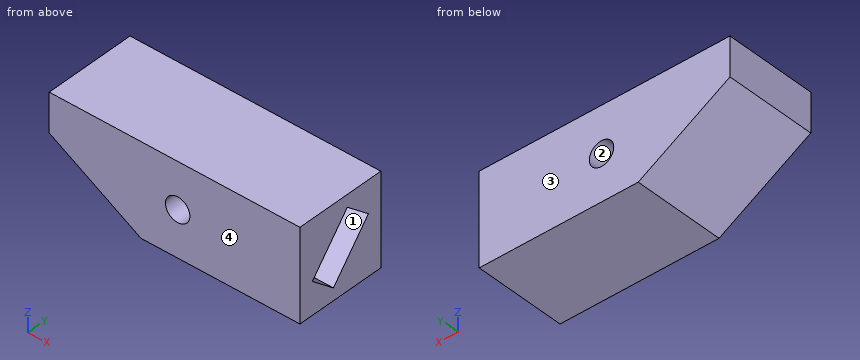
```python
from build123d import *

# Parameters (mm, degrees)
EXTRUDE_1_DEPTH     = 30
SKETCH_2_R          = 4
CUT_EXTRUDE_1_DEPTH = 49.476798574
CUT_EXTRUDE_4_DEPTH = 25
SKETCH1_W           = 30
SKETCH1_H           = 30
BOSS_EXTRUDE1_DEPTH = 27
CHAMFER1_SIZE       = 30
CHAMFER1_SIZE2      = 17.320508076


with BuildPart() as part:
    # Эскиз1 → Бобышка-Вытянуть1 (new body)
    with BuildSketch(Plane(origin=(0, 0, 0), x_dir=(1, 0, 0), z_dir=(0, 1, 0))):
        Polygon((-20, -15), (-35, -15), (-35, 15), (-20, 15), (20, 15), (20, -15), align=None)
    extrude(amount=EXTRUDE_1_DEPTH)

    # Эскиз2 → Вырез-Вытянуть1 (cut, through all)
    with BuildSketch(Plane(origin=(0, 30, 0), x_dir=(1, 0, 0), z_dir=(0, 1, 0))):
        with Locations(Location((-20, 0, 0), (0, 0, 270))):
            Circle(SKETCH_2_R)
    extrude(amount=-CUT_EXTRUDE_1_DEPTH, mode=Mode.SUBTRACT)

    # Эскиз5 → Вырез-Вытянуть4 (cut)
    with BuildSketch(Plane(origin=(20, 0, 0), x_dir=(0, 0, -1), z_dir=(1, 0, 0))):
        Polygon((4.458832066, 4.601018482), (11.015265685, 12.414671802), (-4.458832066, 25.398981518), (-11.015265685, 17.585328198), align=None)
    extrude(amount=-CUT_EXTRUDE_4_DEPTH, mode=Mode.SUBTRACT)

    # Sketch1 → Boss-Extrude1 (add)
    with BuildSketch(Plane.ZY.offset(35)):
        with Locations((0, 15)):
            Rectangle(SKETCH1_W, SKETCH1_H)
    extrude(amount=BOSS_EXTRUDE1_DEPTH)

    # Chamfer1
    chamfer1_edges = [part.edges().sort_by_distance(p)[0] for p in [
        (-62, 15, -15),
    ]]
    chamfer1_side = [part.faces().sort_by_distance(p)[0] for p in [
        (-21, 15, -15),
    ]]
    chamfer(chamfer1_edges, length=CHAMFER1_SIZE, length2=CHAMFER1_SIZE2, reference=chamfer1_side[0])


solid = part.part
```
Verification items for the finished model (mm, model axes). Face numbers are marked on the shaded views. Coordinates: 2 decimals unless noted, no trailing zeros. Loops run counter-clockwise (first coordinate to the right, second up) from the corner with the lowest first, then second, coordinate; pieces in that order, holes last. Notation, with made-up numbers: (57, 39.5) - (85, 39.5) arc R28 cw to (85, 71.5) - close; hole circle Ø10 at (25.25, 1.25). An arc over 180 degrees is marked (long way). Answer as a JSON object with one key per item and string values.
(1) Cross-section at A-A, the plane x = -20. Record the boundary of the cut face in (y, z), then the cut area to 3 significant figures.
Response:
{"outline": "(0, -15) - (30, -15) - (30, -4) - (0, -4) - close; (0, 4) - (30, 4) - (30, 15) - (0, 15) - close", "area": "660 mm²"}
(2) Mould release check, pull along Y, two halves, no side actions. Record for the marked faces 1, 2, 3 and 4: pulls with the +Y half, pulls with the -Y half, needs draft (parallel to the pull), parting line crosses it, or undercut.
Response:
{"face 1": "undercut", "face 2": "needs draft", "face 3": "pulls with the +Y half", "face 4": "pulls with the -Y half"}
(3) Cross-section at D-D, the plane z = 3.25. Record the boundary of the cut face in (x, y).
Response:
{"outline": "(-62, 0) - (-22.33, 0) - (-22.33, 30) - (-62, 30) - close; (-17.67, 0) - (20, 0) - (20, 11.07) - (-5, 11.07) - (-5, 24.38) - (20, 24.38) - (20, 30) - (-17.67, 30) - close"}
(4) Cross-section at B-B, the plane y = 19.75. Record the boundary of the cut face in (x, z).
Response:
{"outline": "(-62, 2.32) - (-32, -15) - (20, -15) - (20, -2.27) - (-5, -2.27) - (-5, 9.2) - (20, 9.2) - (20, 15) - (-62, 15) - close; hole circle Ø8 at (-20, 0)"}
(5) Go/stop test with a flat-tipped pin: pin 1 Ø1 at (x, y) = (-48, 4.5) entering from -Z. Record where the tip stops, or that it passes through.
Response:
{"pin 1": "stops at z = -6.05"}
(6) Cross-section at C-C, the plane x = 3. Record the boundary of the cut face in (y, z), then the cut area to 3 significant figures.
Response:
{"outline": "(0, -15) - (30, -15) - (30, 15) - (0, 15) - close; hole (4.6, -4.46) - (12.41, -11.02) - (25.4, 4.46) - (17.59, 11.02) - close", "area": "694 mm²"}
(7) Scan lines: line 1 along X through (y, z) = (21, 0); line 2 along Z through (x, y) = (8, 8.5); line 3 along X through (y, z) = (13, -1.75). Record each from-to range of solid material in increasing order.
Response:
{"line 1": "x = -57.98 to -24, -16 to -5", "line 2": "z = -15 to -7.73, 0.19 to 15", "line 3": "x = -54.95 to -23.6, -16.4 to -5"}
